Verification items for the finished model (mm, model axes). Face numbers are marked on the shaded views. Round coordinates to 2 decimals unless told otherwise and drop trailing zeros. Order: outer loops, then holes, each group sorted by start corner. A loop starts at its lowest first (then second) coordinate and runs counter-clockwise, first axis right, second up. Notation, with made-up numbers: (-2.5, 77.25) -> (43.5, 77.25) arc R16 cw to (43.5, 85.25) -> close; hole circle Ø5 at (51.5, 1.5). An arc over 180 degrees is marked (long way). Put each result on its own line as item: value.
```python
from build123d import *


with BuildPart() as part:
    # Sketch1 → Revolve1 (revolve)
    with BuildSketch(Plane.XY, mode=Mode.PRIVATE) as revolve1_sk:
        with BuildLine():
            Line((88, 6.5), (56.826927003, 26.292427299))
            Line((56.826927003, 26.292427299), (63.663285359, 26.292427299))
            Line((63.663285359, 26.292427299), (63.663285359, 31.292427299))
            Line((63.663285359, 31.292427299), (48.951927003, 31.292427299))
            Line((48.951927003, 31.292427299), (25, 46.5))
            Line((25, 46.5), (25, 57.273651824))
            Line((25, 57.273651824), (33.5, 57.273651824))
            Line((33.5, 57.273651824), (33.5, 54.773651824))
            Line((33.5, 54.773651824), (28.5, 54.773651824))
            Line((28.5, 54.773651824), (28.5, 48.423651824))
            Line((28.5, 48.423651824), (49.969178626, 34.792427299))
            Line((49.969178626, 34.792427299), (67.163285359, 34.792427299))
            Line((67.163285359, 34.792427299), (67.163285359, 23.875534136))
            Line((67.163285359, 23.875534136), (89.017251622, 10))
            Line((89.017251622, 10), (94.5, 10))
            Line((94.5, 10), (94.5, 6))
            ThreePointArc((94.5, 6), (95.232233047, 4.232233047), (97, 3.5))
            Line((97, 3.5), (100, 3.5))
            Line((100, 3.5), (100, 0))
            Line((100, 0), (97, 0))
            ThreePointArc((97, 0), (92.757359313, 1.757359313), (91, 6))
            Line((91, 6), (91, 6.5))
            Line((91, 6.5), (88, 6.5))
        make_face()
    revolve(revolve1_sk.sketch.rotate(Axis((0, 60.137334415, 0), (0, -1, 0)), 90), axis=Axis((0, 60.137334415, 0), (0, -1, 0)))


solid = part.part
```
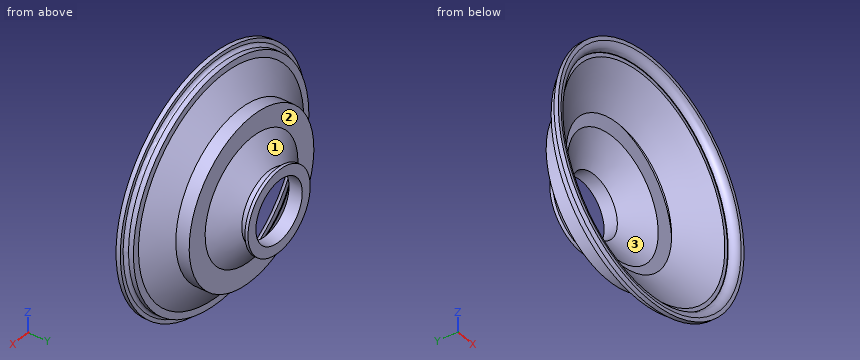
Item 1: Depth check by flat-ended pin: pin 1 Ø10 at (x, z) = (19.5, 75) entering from +Y; pin 2 Ø4 at (y, z) = (10.5, 10) entering from -X; pin 3 Ø12 at (x, z) = (16.5, -34) entering from +Y; pin 4 Ø8 at (x, z) = (-67.5, 45.5) entering from -Y. Enter the tip coordinate at first touch or a pass-through.
Geometry check:
pin 1: y = 20.49
pin 2: x = -94.16
pin 3: y = 57.27
pin 4: y = 8.15
Item 2: Release check for a two-part mould opening along Y. For the marked faces 1, 2 and 3 record: pulls with the +Y half, pulls with the -Y half, needs draft (parallel to the pull), parting line crosses it, or undercut.
Geometry check:
face 1: undercut
face 2: pulls with the +Y half
face 3: pulls with the -Y half
Item 3: Material ranges on line 1 along X through (y, z) = (28.3, 0); line 2 along X through (y, z) = (53.75, 0); line 3 along Z through (x, y) = (6.5, 42), recorded low to high.
Geometry check:
line 1: -67.16 to -63.66, 63.66 to 67.16
line 2: -28.5 to -25, 25 to 28.5
line 3: -38.07 to -31.42, 31.42 to 38.07
Item 4: Sectioned sample at A-A, the plane y = 12.5. Record the boundary of the cut face in (x, z), then the cut area to 3 significant figures.
Geometry check:
outline: circle Ø170.16 at (0, 0); hole circle Ø157.1 at (0, 0)
area: 3,360 mm2
